Can you work these out from the drawing? Everything is in mm from the part's minimum corner. Give positions to 0.01 mm unless a question says otherwise; leave off trailing zeros. Loops run counter-clockwise (first coordinate to the right, second up) from the corner with the lowest first, then second, coordinate; pieces in that order, holes last. Notation, with made-up numbers: (34.5, -29.75) -> (81.5, -29.75) arc R27 cw to (81.5, -11.75) -> close; hole circle Ø1 at (11.5, 9.25). An arc over 180 degrees is marked (long way). Write item = value, one per line. Start each with the question number.
1) I'm going to push flat-ended pins straight in: pin 1 Ø10 at (x, z) = (60.5, 27) entering from -Y; pin 2 Ø3 at (y, z) = (3.5, 12.5) entering from +X (1 decimal); pin 3 Ø6 at (y, z) = (11.5, 17) entering from +X. Where does each tip first touch, or does it pass through?
2) I need wall thicknesses on probe 1 along X at (y, z) = (2.25, 18.5); probe 2 along Z at (x, y) = (25, 13.75); probe 3 along Z at (x, y) = (18, 11.75). Which ranges of each line are inside material? Lowest first, please. Write a range as from..to.
3) I want a section at B-B (z = 25.5). List the corners of the cut face in (x, y) for me.
4) I want a section at A-A (y = 5). List the corners of the cut face in (x, z) for me, and give its area (3 significant figures).
5) I want a section at C-C (x = 68). List the corners of the cut face in (y, z) for me, and give its area (3 significant figures).
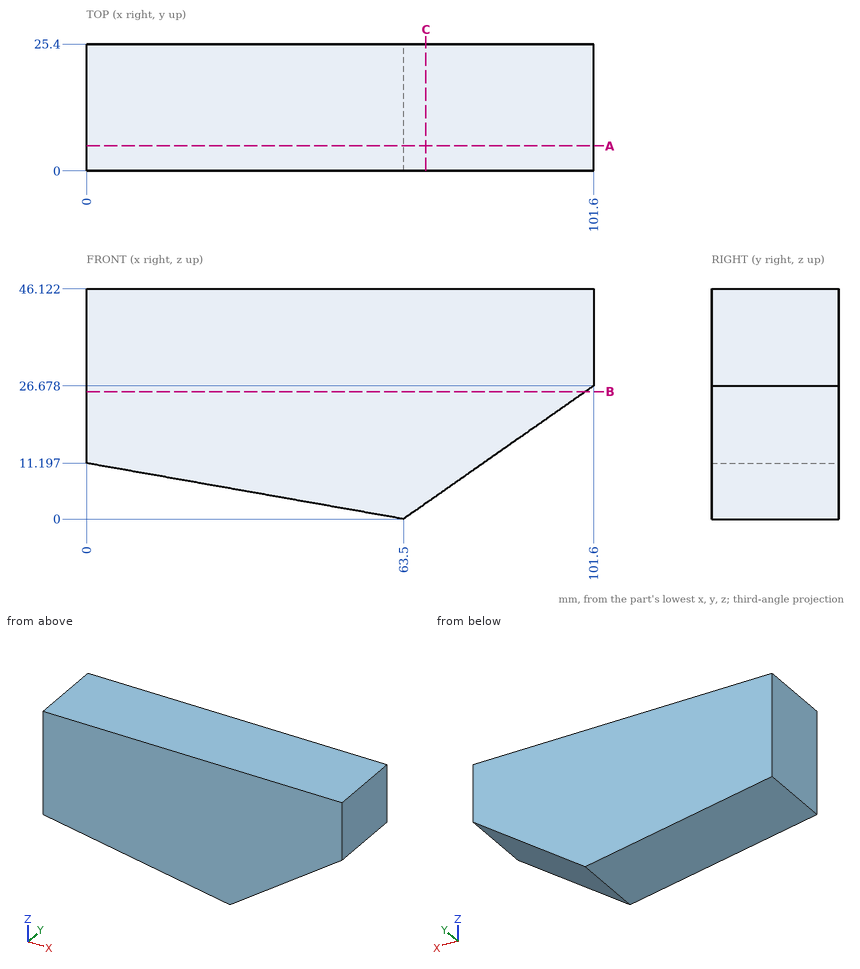
Answer list:
q1.pin_1 = 0
q1.pin_2 = 83.5
q1.pin_3 = 92.06
q2.probe_1 = 0..89.92
q2.probe_2 = 6.79..46.12
q2.probe_3 = 8.02..46.12
q3.outline = (0, 0) -> (99.92, 0) -> (99.92, 25.4) -> (0, 25.4) -> close
q4.outline = (0, 11.2) -> (63.5, 0) -> (101.6, 26.68) -> (101.6, 46.12) -> (0, 46.12) -> close
q4.area = 3,820 mm^2
q5.outline = (0, 3.15) -> (25.4, 3.15) -> (25.4, 46.12) -> (0, 46.12) -> close
q5.area = 1,090 mm^2
